```python
from build123d import *

# Parameters (mm, degrees)
BOSS_EXTRUDE1_DEPTH = 2.54
SKETCH3_W           = 25.4
SKETCH3_H           = 12.7
SKETCH3_W_2         = 20.32
SKETCH3_H_2         = 7.62
BOSS_EXTRUDE3_DEPTH = 2.54
SKETCH4_R           = 1.905
BOSS_EXTRUDE4_DEPTH = 5.08
SKETCH5_R           = 3.81
SKETCH5_R_2         = 1.5
BOSS_EXTRUDE5_DEPTH = 2.54
SKETCH6_W           = 25.4
SKETCH6_H           = 12.7
SKETCH6_W_2         = 20.32
SKETCH6_H_2         = 7.62
BOSS_EXTRUDE8_DEPTH = 2.54
SKETCH12_W          = 5
SKETCH12_H          = 5
CUT_EXTRUDE1_DEPTH  = 2.54


with BuildPart() as part:
    # Sketch2 → Boss-Extrude1 (new body)
    with BuildSketch(Plane(origin=(0, 0, 0), x_dir=(1, 0, 0), z_dir=(0, 1, 0))):
        Polygon((-80.183865598, 25.601069918), (48.816134402, 27.536069918), (48.816134402, -18.304155069), (-80.183865598, -16.369155069), align=None)
    extrude(amount=BOSS_EXTRUDE1_DEPTH)

    # Sketch3 → Boss-Extrude3 (add)
    # profile 1 of 2: a face of its own
    with BuildSketch(Plane(origin=(0.046703878, 0, 17.572613611), x_dir=(0.9998875189808162, 0, 0.014998312784712321), z_dir=(-0.01499831278471232, 0, 0.9998875189808161))):
        with Locations((-54.839594907, -3.81)):
            Rectangle(SKETCH3_W, SKETCH3_H)
        with Locations((-54.839594907, -3.81)):
            Rectangle(SKETCH3_W_2, SKETCH3_H_2, mode=Mode.SUBTRACT)
    # profile 2 of 2: a face of its own
    with BuildSketch(Plane(origin=(0.046703878, 0, 17.572613611), x_dir=(0.9998875189808162, 0, 0.014998312784712321), z_dir=(-0.01499831278471232, 0, 0.9998875189808161))):
        with Locations((23.374916777, -3.81)):
            Rectangle(SKETCH3_W, SKETCH3_H)
        with Locations((23.374916777, -3.81)):
            Rectangle(SKETCH3_W_2, SKETCH3_H_2, mode=Mode.SUBTRACT)
    extrude(amount=BOSS_EXTRUDE3_DEPTH)

    # Sketch4 → Boss-Extrude4 (add)
    with BuildSketch(Plane.XZ):
        with Locations(Location((-72.563865598, 8.982611367, 0), (0, 0, 270))):
            Circle(SKETCH4_R)
        with Locations(Location((-72.183865598, -18.220226216, 0), (0, 0, 270))):
            Circle(SKETCH4_R)
        with Locations(Location((41.196134402, -19.920926216, 0), (0, 0, 270))):
            Circle(SKETCH4_R)
        with Locations(Location((41.196134402, 10.689011367, 0), (0, 0, 270))):
            Circle(SKETCH4_R)
    extrude(amount=BOSS_EXTRUDE4_DEPTH)

    # Sketch5 → Boss-Extrude5 (add)
    # profile 1 of 4: a face of its own
    with BuildSketch(Plane(origin=(0, 2.54, 0), x_dir=(1, 0, 0), z_dir=(0, 1, 0))):
        with Locations(Location((-70.023865598, 17.115957425, 0), (0, 0, 90))):
            Circle(SKETCH5_R)
        with Locations(Location((-70.023865598, 17.115957425, 0), (0, 0, 270))):
            Circle(SKETCH5_R_2, mode=Mode.SUBTRACT)
    # profile 2 of 4: a face of its own
    with BuildSketch(Plane(origin=(0, 2.54, 0), x_dir=(1, 0, 0), z_dir=(0, 1, 0))):
        with Locations(Location((-70.023865598, -7.884042575, 0), (0, 0, 90))):
            Circle(SKETCH5_R)
        with Locations(Location((-70.023865598, -7.884042575, 0), (0, 0, 270))):
            Circle(SKETCH5_R_2, mode=Mode.SUBTRACT)
    # profile 3 of 4: a face of its own
    with BuildSketch(Plane(origin=(0, 2.54, 0), x_dir=(1, 0, 0), z_dir=(0, 1, 0))):
        with Locations(Location((38.656134402, -7.884042575, 0), (0, 0, 90))):
            Circle(SKETCH5_R)
        with Locations(Location((38.656134402, -7.884042575, 0), (0, 0, 270))):
            Circle(SKETCH5_R_2, mode=Mode.SUBTRACT)
    # profile 4 of 4: a face of its own
    with BuildSketch(Plane(origin=(0, 2.54, 0), x_dir=(1, 0, 0), z_dir=(0, 1, 0))):
        with Locations(Location((38.656134402, 17.115957425, 0), (0, 0, 90))):
            Circle(SKETCH5_R)
        with Locations(Location((38.656134402, 17.115957425, 0), (0, 0, 270))):
            Circle(SKETCH5_R_2, mode=Mode.SUBTRACT)
    extrude(amount=BOSS_EXTRUDE5_DEPTH)

    # Sketch6 → Boss-Extrude8 (add)
    # profile 1 of 2: a face of its own
    with BuildSketch(Plane(origin=(-0.401966976, 0, -26.797798398), x_dir=(-0.9998875189808162, 0, 0.014998312784712349), z_dir=(-0.014998312784712347, 0, -0.9998875189808161))):
        with Locations((-23.097259161, -3.81)):
            Rectangle(SKETCH6_W, SKETCH6_H)
        with Locations((-23.097259161, -3.81)):
            Rectangle(SKETCH6_W_2, SKETCH6_H_2, mode=Mode.SUBTRACT)
    # profile 2 of 2: a face of its own
    with BuildSketch(Plane(origin=(-0.401966976, 0, -26.797798398), x_dir=(-0.9998875189808162, 0, 0.014998312784712349), z_dir=(-0.014998312784712347, 0, -0.9998875189808161))):
        with Locations((54.390873581, -3.81)):
            Rectangle(SKETCH6_W, SKETCH6_H)
        with Locations((54.390873581, -3.81)):
            Rectangle(SKETCH6_W_2, SKETCH6_H_2, mode=Mode.SUBTRACT)
    extrude(amount=BOSS_EXTRUDE8_DEPTH)

    # Sketch12 → Cut-Extrude1 (cut)
    with BuildSketch(Plane(origin=(0, 2.54, 0), x_dir=(1, 0, 0), z_dir=(0, 1, 0))):
        with Locations((-50.183865598, 15.131238659)):
            Rectangle(SKETCH12_W, SKETCH12_H)
        with Locations((-50.183865598, 8.131238659)):
            Rectangle(SKETCH12_W, SKETCH12_H)
        with Locations((-15.183865598, 22.10067619)):
            Rectangle(SKETCH12_W, SKETCH12_H)
        with Locations((-15.183865598, 15.131238659)):
            Rectangle(SKETCH12_W, SKETCH12_H)
        with Locations((-15.183865598, 8.131238659)):
            Rectangle(SKETCH12_W, SKETCH12_H)
        with Locations((-15.183865598, 1.131238659)):
            Rectangle(SKETCH12_W, SKETCH12_H)
        with Locations((-15.183865598, -5.868761341)):
            Rectangle(SKETCH12_W, SKETCH12_H)
        with Locations((14.816134346, -12.868761341)):
            Rectangle(SKETCH12_W, SKETCH12_H)
        with Locations((14.816134346, -5.868761341)):
            Rectangle(SKETCH12_W, SKETCH12_H)
        with Locations((14.816134346, 22.10067619)):
            Rectangle(SKETCH12_W, SKETCH12_H)
        with Locations((14.816134346, 15.131238659)):
            Rectangle(SKETCH12_W, SKETCH12_H)
    extrude(amount=-CUT_EXTRUDE1_DEPTH, mode=Mode.SUBTRACT)


solid = part.part
```
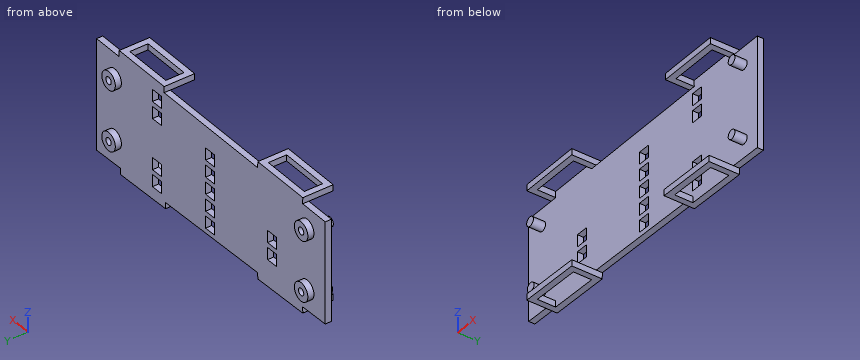
Geometry check sheet. Reference: the model listing, model coordinates, mm. Give positions to 0.01 mm unless a question says otherwise; leave off trailing zeros. Order: outer loops, then holes, each group sorted by start corner. A loop starts at its lowest first (then second) coordinate and runs counter-clockwise, first axis right, second up. Notation, with made-up numbers: (63.25, 76) -> (103.25, 76) arc R14 ccw to (103.25, 101) -> close; hole circle Ø2 at (17.5, 4.5). An arc over 180 degrees is marked (long way). Write each question's results on one line, items separated by ' | '. Start each with the question number.
(1) Sectioned sample at B-B (x = 15.5). Enter the section's corners in (y, z).
(2) Sectioned sample at A-A (z = -1.5). Enter the section's corners in (x, y), plus the area to 3 significant figures.
(3) Scan lines: line 1 (Z direction, x = 38, y = 3); line 2 (X direction, y = 1.75, z = 14); line 3 (Y direction, x = -57, z = -9). Record each from-to range of solid material in increasing order.
(4) Sectioned sample at C-C (x = -55). Enter the section's corners in (y, z).
(5) Gauge pin test, flat ends, axial feed: P1, Ø3, axis at x = 15.5, y = 1, coming from the +Z side; P2, Ø5, axis at x = -4.5, y = 1.5, coming from the +Z side; P3, Ø2, axis at y = -5.5, z = 8.5, coming from the +X side. Record the tip position at first contact, or that the pin passes through.
(6) Sectioned sample at D-D (y = -2). Give the number of separate pieces and of enclosed holes in the cut face, plus the area to 3 significant figures.
Answer below:
1) outline: (-10.16, -29.58) -> (-7.62, -29.58) -> (-7.62, -27.04) -> (-10.16, -27.04) -> close; (-10.16, 17.8) -> (-7.62, 17.8) -> (-7.62, 20.34) -> (-10.16, 20.34) -> close; (0, -29.58) -> (2.54, -29.58) -> (2.54, -24.6) -> (0, -24.6) -> close; (0, -19.6) -> (2.54, -19.6) -> (2.54, -17.63) -> (0, -17.63) -> close; (0, -12.63) -> (2.54, -12.63) -> (2.54, 3.37) -> (0, 3.37) -> close; (0, 8.37) -> (2.54, 8.37) -> (2.54, 10.37) -> (0, 10.37) -> close; (0, 15.37) -> (2.54, 15.37) -> (2.54, 20.34) -> (0, 20.34) -> close
2) outline: (-80.18, 0) -> (-17.68, 0) -> (-17.68, 2.54) -> (-80.18, 2.54) -> close; (-12.68, 0) -> (48.82, 0) -> (48.82, 2.54) -> (-12.68, 2.54) -> close | area: 315 mm2
3) line 1: -20.87 to -18.46, -15.77 to -13.36, 4.13 to 6.54, 9.23 to 11.64 | line 2: -80.18 to 12.32, 17.32 to 48.82 | line 3: 0 to 2.54
4) outline: (-10.16, -28.52) -> (-7.62, -28.52) -> (-7.62, -25.98) -> (-10.16, -25.98) -> close; (-10.16, 16.75) -> (-7.62, 16.75) -> (-7.62, 19.29) -> (-10.16, 19.29) -> close; (0, -28.52) -> (2.54, -28.52) -> (2.54, 19.29) -> (0, 19.29) -> close
5) P1: z = 20.37 | P2: z = 17.54 | P3: x = 42.61
6) separate pieces: 12 | enclosed holes: 0 | area: 97.2 mm2
